Input: part model. Units: mm. Frame: model coordinates. A direction names the side the tool comes from. Give positions to 0.01 mm unless a question says otherwise; leave off trailing zeros. Order: outer loops, then holes, each group sorted by start corner. A loop starts at its lowest first (then second) coordinate and runs counter-clockwise, first axis right, second up. Notation, with made-up numbers: (-17, 13.5) - (41, 13.5) arc R23 ccw to (41, 44.5) - close; hole circle Ø7 at (46.25, 77.5). An arc over 180 degrees is marked (long way). Use a Markdown table: item, result.
from build123d import *

# Parameters (mm, degrees)
SKETCH1_R           = 1.5
SKETCH1_R_2         = 0.5
BOSS_EXTRUDE1_DEPTH = 0.8
SKETCH2_W           = 4
SKETCH2_H           = 5
BOSS_EXTRUDE2_DEPTH = 2


with BuildPart() as part:
    # Sketch1 → Boss-Extrude1 (new body, symmetric)
    with BuildSketch(Plane.XY):
        with BuildLine():
            Line((-8.5, -11.5), (8.5, -11.5))
            ThreePointArc((8.5, -11.5), (10.621320344, -10.621320344), (11.5, -8.5))
            Line((11.5, -8.5), (11.5, 8.5))
            ThreePointArc((11.5, 8.5), (10.621320344, 10.621320344), (8.5, 11.5))
            Line((8.5, 11.5), (-8.5, 11.5))
            ThreePointArc((-8.5, 11.5), (-10.621320344, 10.621320344), (-11.5, 8.5))
            Line((-11.5, 8.5), (-11.5, -8.5))
            ThreePointArc((-11.5, -8.5), (-10.621320344, -10.621320344), (-8.5, -11.5))
        make_face()
        with Locations((-8, 8)):
            Circle(SKETCH1_R, mode=Mode.SUBTRACT)
        with Locations((8, 8)):
            Circle(SKETCH1_R, mode=Mode.SUBTRACT)
        with Locations((8, -8)):
            Circle(SKETCH1_R, mode=Mode.SUBTRACT)
        with Locations((-8, -8)):
            Circle(SKETCH1_R, mode=Mode.SUBTRACT)
        with Locations((0, -8)):
            Circle(SKETCH1_R_2, mode=Mode.SUBTRACT)
        with Locations((-2.54, -8)):
            Circle(SKETCH1_R_2, mode=Mode.SUBTRACT)
        with Locations((2.54, -8)):
            Circle(SKETCH1_R_2, mode=Mode.SUBTRACT)
        with Locations((-1.27, 8)):
            Circle(SKETCH1_R_2, mode=Mode.SUBTRACT)
        with Locations((1.27, 8)):
            Circle(SKETCH1_R_2, mode=Mode.SUBTRACT)
        with Locations((-3.81, 8)):
            Circle(SKETCH1_R_2, mode=Mode.SUBTRACT)
        with Locations((3.81, 8)):
            Circle(SKETCH1_R_2, mode=Mode.SUBTRACT)
    extrude(amount=BOSS_EXTRUDE1_DEPTH, both=True)

    # Sketch2 → Boss-Extrude2 (add)
    with BuildSketch(Plane.XY.offset(0.8)):
        Rectangle(SKETCH2_W, SKETCH2_H)
    extrude(amount=BOSS_EXTRUDE2_DEPTH)


solid = part.part
1. Material intervals for line 1 along Y through (x, z) = (8, -0.25); line 2 along Y through (x, z) = (2.54, 0.2); line 3 along Y through (x, z) = (-3.81, 0), sorted ascending.
Response:
| item | result |
|---|---|
| line 1 | y = -11.5 to -9.5, -6.5 to 6.5, 9.5 to 11.5 |
| line 2 | y = -11.5 to -8.5, -7.5 to 11.5 |
| line 3 | y = -11.5 to 7.5, 8.5 to 11.5 |
2. Section query B-B (z = 0.5). State how many separate pieces and enclosed holes the cut face has, then the cut area to 3 significant figures.
Response:
| item | result |
|---|---|
| separate pieces | 1 |
| enclosed holes | 11 |
| area | 488 mm^2 |
3. Set-up query: faces 4 (the face through (-2, 0, 2)), 5 (the face through (-0.108, -8.488, -0.011)). Return all of +Z, -Z, +X, -X, +Y, -Y with unobstructed straight access to the full face (end or side cutting, diameter ignored); none if empty.
Response:
| item | result |
|---|---|
| face 4 | +Z, -X, +Y, -Y |
| face 5 | +Z, -Z |
4. Pin query (flat end, axial travel): pin 1 (5 mm diameter, centred on x = 3, y = 4, fed in from +Z); pin 2 (1 mm diameter, centred on y = 0.5, z = 1.5, fed in from -X); pin 3 (0.6 mm diameter, centred on x = 0.5, z = 2, fed in from +Y); pin 4 (5 mm diameter, centred on x = 8, y = 8, fed in from +Z). Return the tip coordinate at first contact, or that it passes through.
Response:
| item | result |
|---|---|
| pin 1 | stops at z = 2.8 |
| pin 2 | stops at x = -2 |
| pin 3 | stops at y = 2.5 |
| pin 4 | stops at z = 0.8 |
5. Section query A-A (x = 2.54). Return loops of the section in (y, z).
Response:
| item | result |
|---|---|
| outline | (-11.5, -0.8) - (-8.5, -0.8) - (-8.5, 0.8) - (-11.5, 0.8) - close; (-7.5, -0.8) - (11.5, -0.8) - (11.5, 0.8) - (-7.5, 0.8) - close |
6. Section query C-C (y = 8). Return loops of the section in (x, z).
Response:
| item | result |
|---|---|
| outline | (-11.5, -0.8) - (-9.5, -0.8) - (-9.5, 0.8) - (-11.5, 0.8) - close; (-6.5, -0.8) - (-4.31, -0.8) - (-4.31, 0.8) - (-6.5, 0.8) - close; (-3.31, -0.8) - (-1.77, -0.8) - (-1.77, 0.8) - (-3.31, 0.8) - close; (-0.77, -0.8) - (0.77, -0.8) - (0.77, 0.8) - (-0.77, 0.8) - close; (1.77, -0.8) - (3.31, -0.8) - (3.31, 0.8) - (1.77, 0.8) - close; (4.31, -0.8) - (6.5, -0.8) - (6.5, 0.8) - (4.31, 0.8) - close; (9.5, -0.8) - (11.5, -0.8) - (11.5, 0.8) - (9.5, 0.8) - close |
7. Mould query, pull axis X, two halves, no side actions, for faces 1 (the face through (0, 2.5, 2)), 2 (the face through (6.8, 7.1, 0)), 3 (the face through (2, 0, 2)). Classes: pulls with the +X half, pulls with the -X half, needs draft (parallel to the pull), parting line crosses it, or undercut.
Response:
| item | result |
|---|---|
| face 1 | needs draft |
| face 2 | undercut |
| face 3 | pulls with the +X half |
8. Section query D-D (x = -8). Return loops of the section in (y, z), then the cut area to 3 significant figures.
Response:
| item | result |
|---|---|
| outline | (-11.5, -0.8) - (-9.5, -0.8) - (-9.5, 0.8) - (-11.5, 0.8) - close; (-6.5, -0.8) - (6.5, -0.8) - (6.5, 0.8) - (-6.5, 0.8) - close; (9.5, -0.8) - (11.5, -0.8) - (11.5, 0.8) - (9.5, 0.8) - close |
| area | 27.2 mm^2 |
